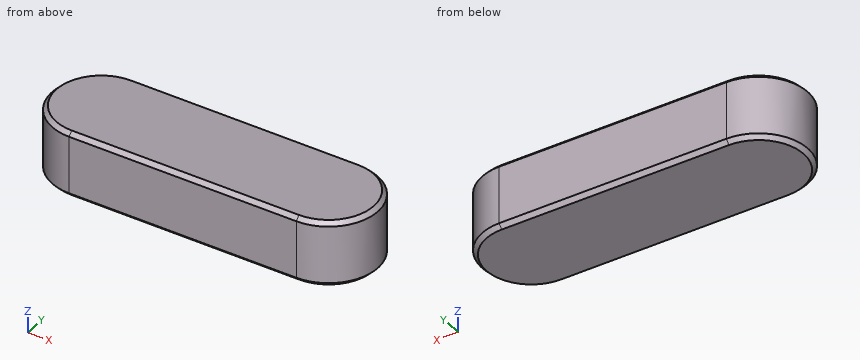
```python
from build123d import *

# Parameters (mm, degrees)
EXTRUDE1_DEPTH = 4
CHAMFER1_SIZE  = 0.25


with BuildPart() as part:
    # Sketch1 → Extrude1 (new body)
    with BuildSketch(Plane.XY):
        with BuildLine():
            Line((0, 3), (-14, 3))
            ThreePointArc((-14, 3), (-17, 0), (-14, -3))
            Line((-14, -3), (0, -3))
            ThreePointArc((0, -3), (3, 0), (0, 3))
        make_face()
    extrude(amount=EXTRUDE1_DEPTH)

    # Chamfer1
    chamfer1_edges = [part.edges().sort_by_distance(p)[0] for p in [
        (-17, 0, 4),
        (-7, -3, 4),
        (3, 0, 4),
        (-7, -3, 0),
        (-17, 0, 0),
        (-7, 3, 0),
        (3, 0, 0),
        (-7, 3, 4),
    ]]
    chamfer(chamfer1_edges, length=CHAMFER1_SIZE)


solid = part.part
```
Check sheet for the modelled part. Datum: model origin and axes. Units: mm. Coordinates: 2 decimals unless noted, no trailing zeros. Order: outer loops, then holes, each group sorted by start corner. A loop starts at its lowest first (then second) coordinate and runs counter-clockwise, first axis right, second up. Notation, with made-up numbers: M 89,17 L 116,17 A19 cw 116,34 Z; hole C -13,84 d9. An arc over 180 degrees is marked long. Write each question's results on one line, items separated by ' | '. Start each with the question number.
1. Cross-section at A-A on z = 1.2. Record the cut outline in (x, y), and give its area (3 significant figures).
2. Material ranges on probe 1 along Y at (x, z) = (-12.5, 3.85); probe 2 along X at (y, z) = (2, 2.25); probe 3 along X at (y, z) = (0.75, 2.1), recorded low to high.
3. Go/stop test with a flat-tipped pin: P1, Ø1.5, axis at y = -1, z = 2.5, coming from the -X side. Record where the tip stops, or that it passes through.
Checks:
1) outline: M -14,-3 L 0,-3 A3 ccw 0,3 L -14,3 A3 ccw Z | area: 112 mm²
2) probe 1: y = -2.9 to 2.9 | probe 2: x = -16.24 to 2.24 | probe 3: x = -16.9 to 2.9
3) P1: stops at x = -16.99
